Read the model definition and answer for the solid it produces. Units are mm, in the model's axes. Give positions to 0.01 mm unless a question says otherwise; leave off trailing zeros. Order: outer loops, then holes, each group sorted by start corner. A loop starts at its lowest first (then second) coordinate and runs counter-clockwise, first axis right, second up. Notation, with made-up numbers: (44, 54.25) - (61, 54.25) arc R28 ccw to (61, 88.25) - close; hole circle Ø2 at (-36.75, 24). An arc over 180 degrees is marked (long way). Write each question's results on one line, items separated by ' | '. Start each with the question number.
Q1. A flat-ended cylindrical pin translates along its axis: P1, Ø0.6, axis at x = -28.5, y = 1, coming from the -Z side. Find the tip coordinate at first contact, or state that the pin passes through.
Q2. Find section B-B on z = -5. Give the vertices of the cut face in (x, y).
Q3. Find the intervals of material crossed by line 1 along Z through (x, y) = (-25, 0.1); line 2 along Z through (x, y) = (-34.5, 0.55); line 3 along X through (y, z) = (1.2, -2), in increasing order. Write a range as from..to.
from build123d import *

# Parameters (mm, degrees)
EXTRUDE_1_DEPTH     = 2
SKETCH_2_W          = 12
SKETCH_2_H          = 1
CUT_EXTRUDE_1_DEPTH = 2
FILLET_1_R          = 1
FILLET_2_R          = 1


with BuildPart() as part:
    # 草图1 → 凸台-拉伸1 (new body)
    with BuildSketch(Plane(origin=(0, 0, 0), x_dir=(1, 0, 0), z_dir=(0, 1, 0))):
        Polygon((-40, 11), (-40, 40), (40, 40), (40, -40), (-40, -40), (-40, -11), (-34, -11), (-34, 11), align=None)
    extrude(amount=EXTRUDE_1_DEPTH)

    # 草图2 → 切除-拉伸1 (cut)
    with BuildSketch(Plane(origin=(0, 2, 0), x_dir=(1, 0, 0), z_dir=(0, 1, 0))):
        with Locations((-28, 39.5)):
            Rectangle(SKETCH_2_W, SKETCH_2_H)
        with Locations((28, 39.5)):
            Rectangle(SKETCH_2_W, SKETCH_2_H)
    extrude(amount=-CUT_EXTRUDE_1_DEPTH, mode=Mode.SUBTRACT)

    # 圆角1
    fillet_1_edges = [part.edges().sort_by_distance(p)[0] for p in [
        (22, 1, -39),
        (34, 1, -39),
        (-34, 1, -39),
        (-22, 1, -39),
    ]]
    fillet(fillet_1_edges, radius=FILLET_1_R - 0.0001)  # a hair under: the kernel refuses the full size

    # 圆角2
    fillet_2_edges = [part.edges().sort_by_distance(p)[0] for p in [
        (-34, 1, 11),
        (-34, 1, -11),
    ]]
    fillet(fillet_2_edges, radius=FILLET_2_R)


solid = part.part
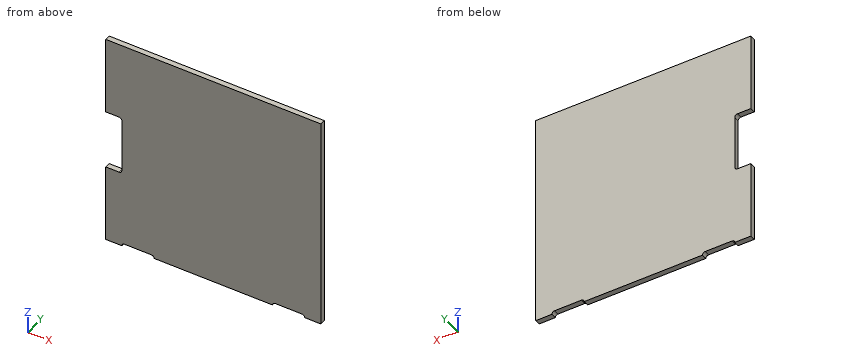
Working result:
1) P1: z = -39
2) outline: (-34, 0) - (40, 0) - (40, 2) - (-34, 2) - close
3) line 1: -39..40 | line 2: -40..-10.87, 10.87..40 | line 3: -34..40
